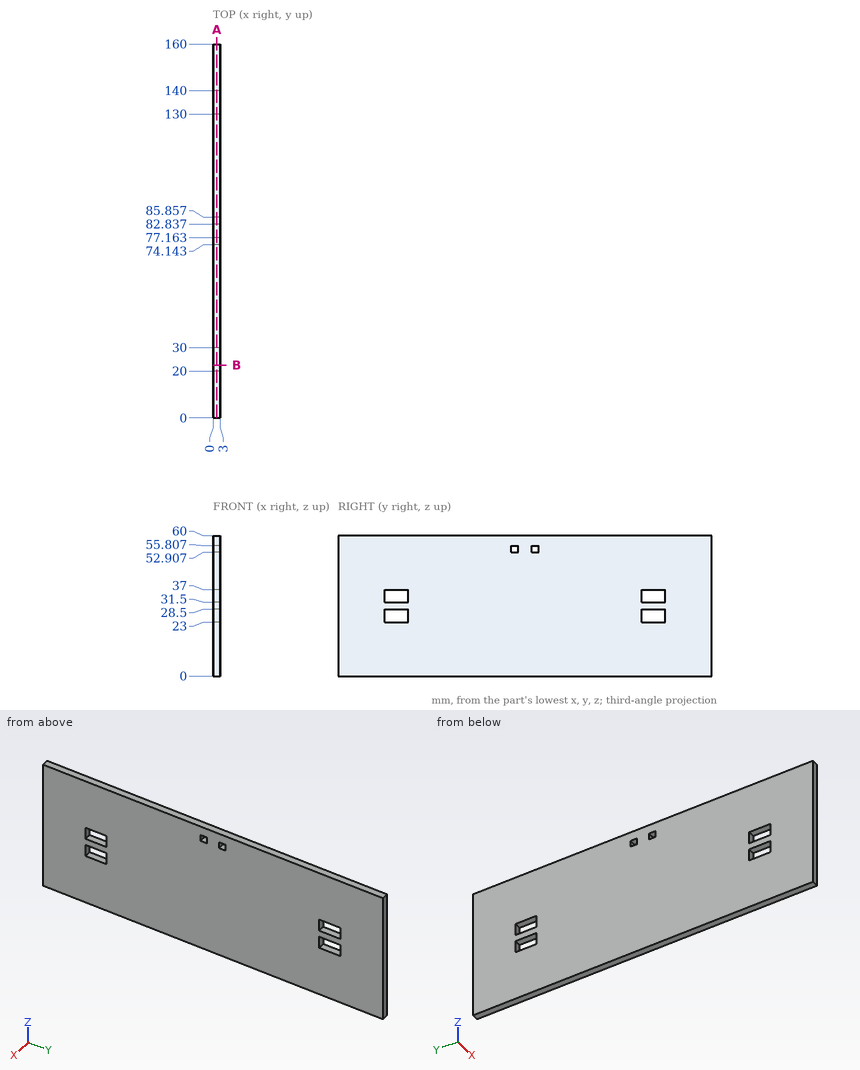
Print and shaded views of the part. All mm, measured from the part's lowest x, y and z. Give positions to 0.01 mm unless a question says otherwise; leave off trailing zeros. Loops run counter-clockwise (first coordinate to the right, second up) from the corner with the lowest first, then second, coordinate; pieces in that order, holes last. Notation, with made-up numbers: (80.5, 50) -> (107.5, 50) arc R10 ccw to (107.5, 59) -> close; hole circle Ø9 at (-24.5, 62.5). An arc over 180 degrees is marked (long way). Use a Markdown table: item, result.
1. Wall check: L1, parallel to Z at x = 0.95, y = 133; L2, parallel to Y at x = 0.75, z = 26.5; L3, parallel to Z at x = 1.45, y = 75.5. Give the ranges that are in metal, low to high. Write a range as [from, to].
Check result:
| item | result |
|---|---|
| L1 | z = [0, 23], [28.5, 31.5], [37, 60] |
| L2 | y = [0, 20], [30, 130], [140, 160] |
| L3 | z = [0, 52.91], [55.81, 60] |
2. Slice it at B-B (y = 22.5). List the corners of the cut face in (x, z).
Check result:
| item | result |
|---|---|
| outline | (0, 0) -> (3, 0) -> (3, 23) -> (0, 23) -> close; (0, 28.5) -> (3, 28.5) -> (3, 31.5) -> (0, 31.5) -> close; (0, 37) -> (3, 37) -> (3, 60) -> (0, 60) -> close |
3. Slice it at A-A (x = 1.6). List the corners of the cut face in (y, z).
Check result:
| item | result |
|---|---|
| outline | (0, 0) -> (160, 0) -> (160, 60) -> (0, 60) -> close; hole (20, 23) -> (30, 23) -> (30, 28.5) -> (20, 28.5) -> close; hole (20, 31.5) -> (30, 31.5) -> (30, 37) -> (20, 37) -> close; hole (74.14, 52.91) -> (77.16, 52.91) -> (77.16, 55.81) -> (74.14, 55.81) -> close; hole (82.84, 52.91) -> (85.86, 52.91) -> (85.86, 55.81) -> (82.84, 55.81) -> close; hole (130, 23) -> (140, 23) -> (140, 28.5) -> (130, 28.5) -> close; hole (130, 31.5) -> (140, 31.5) -> (140, 37) -> (130, 37) -> close |
